For this review, use the dimensioned drawing (mm, ordinates from the lowest corner) and the shaded views. A direction names the side the tool comes from. Give positions to 0.01 mm unless a question says otherwise; leave off trailing zeros. Loops run counter-clockwise (first coordinate to the right, second up) from the corner with the lowest first, then second, coordinate; pieces in that order, holes last. Notation, with made-up numbers: (-22, -25.5) -> (10, -25.5) arc R32 ccw to (10, 3.5) -> close; hole circle Ø11 at (83.5, 26.25). An arc over 180 degrees is marked (long way). Use a Markdown table: item, result. Add a question column.
1. For pin 1 Ø6 at (y, z) = (65.5, 10.5) entering from +X; pin 2 Ø5 at (y, z) = (22, 82.5) entering from +X, all flat-tipped, find the tip position at first contact; note any pin that passes through.
2. To check wall thickness, follow line 1 (Y direction, x = 22, z = 4); line 2 (Z direction, x = 37, y = 32.5); line 3 (Z direction, x = 102, y = 17.5). State the ranges of each line that lie inside material, in increasing order.
3. Add section B-B (x = 87). State the section outline as (y, z) points.
4. Add section A-A (x = 22.5). State the section outline as (y, z) points.
5. For the marked faces 4, 5 and 6, list the 3-axis set-ups (+Z, -Z, +X, -X, +Y, -Y) from which the entire face can be reached by the end or side of a thin tool; tool diameter is ignored.
6. Add section D-D (y = 40). State the section outline as (x, z) points, and give its area (3 significant figures).
7. Add section C-C (y = 76.5). State the section outline as (x, z) points.
8. Draft analysis for pull direction X (two halves, no side actions). For the marked faces 1, 2 and 3, state which applies: pulls with the +X half, pulls with the -X half, needs draft (parallel to the pull), parting line crosses it, or undercut.
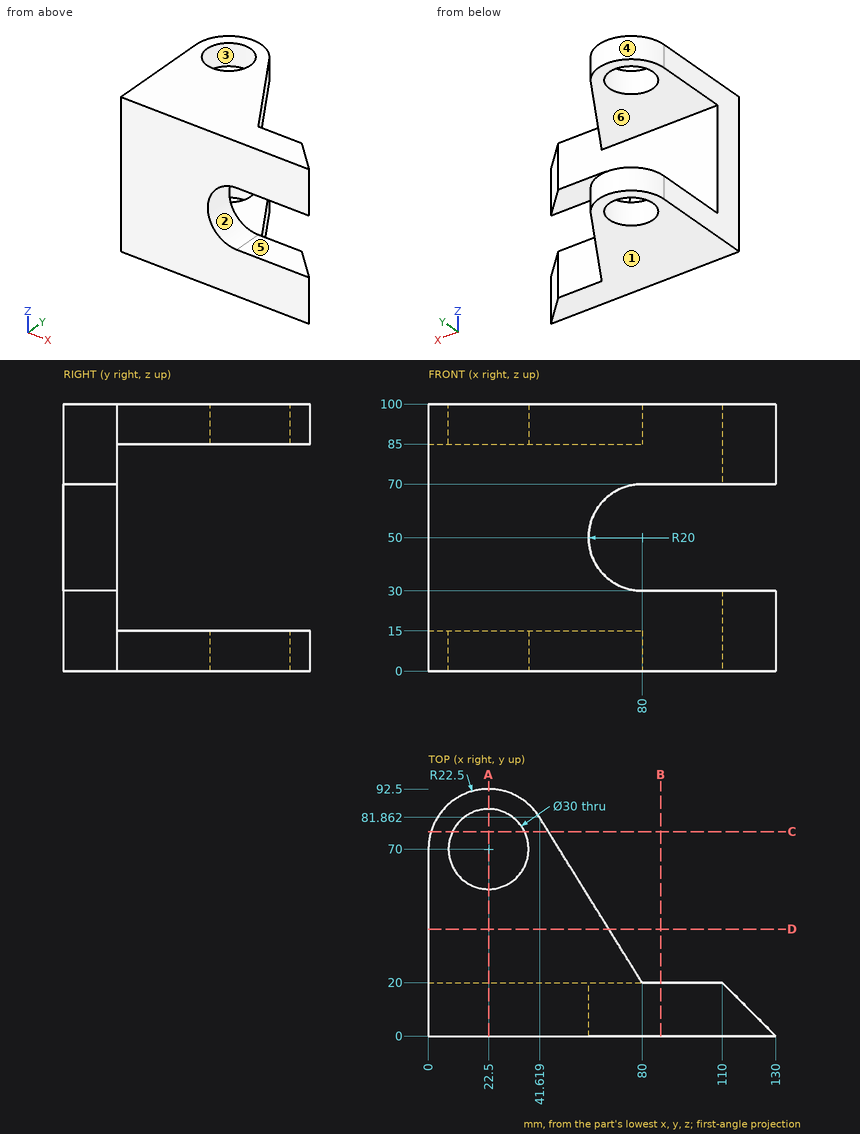
Taken from the geometry:
| question | item | result |
|---|---|---|
| 1 | pin 1 | stops at x = 53.63 |
| 1 | pin 2 | stops at x = 110.5 |
| 2 | line 1 | y = 0 to 55.01, 84.99 to 92.49 |
| 2 | line 2 | z = 0 to 15, 85 to 100 |
| 2 | line 3 | z = 0 to 30, 70 to 100 |
| 3 | outline | (0, 0) -> (20, 0) -> (20, 30) -> (0, 30) -> close; (0, 70) -> (20, 70) -> (20, 100) -> (0, 100) -> close |
| 4 | outline | (0, 0) -> (55, 0) -> (55, 15) -> (20, 15) -> (20, 85) -> (55, 85) -> (55, 100) -> (0, 100) -> close; (85, 0) -> (92.5, 0) -> (92.5, 15) -> (85, 15) -> close; (85, 85) -> (92.5, 85) -> (92.5, 100) -> (85, 100) -> close |
| 5 | face 4 | +Z, -Z, +Y |
| 5 | face 5 | +X, +Y, -Y |
| 5 | face 6 | +X, -X, +Y |
| 6 | outline | (0, 0) -> (67.59, 0) -> (67.59, 15) -> (0, 15) -> close; (0, 85) -> (67.59, 85) -> (67.59, 100) -> (0, 100) -> close |
| 6 | area | 2,030 mm^2 |
| 7 | outline | (0.96, 0) -> (8.98, 0) -> (8.98, 15) -> (0.96, 15) -> close; (0.96, 85) -> (8.98, 85) -> (8.98, 100) -> (0.96, 100) -> close; (36.02, 0) -> (44.95, 0) -> (44.95, 15) -> (36.02, 15) -> close; (36.02, 85) -> (44.95, 85) -> (44.95, 100) -> (36.02, 100) -> close |
| 8 | face 1 | needs draft |
| 8 | face 2 | pulls with the +X half |
| 8 | face 3 | undercut |
